Could you check a few things on this model? Use its own coordinates, in mm. Round coordinates to 2 decimals unless told otherwise and drop trailing zeros. Loops run counter-clockwise (first coordinate to the right, second up) from the corner with the lowest first, then second, coordinate; pieces in that order, holes last. Notation, with made-up numbers: (11.5, -38.5) - (37.5, -38.5) arc R15 ccw to (37.5, -22.5) - close; hole circle Ø1 at (-20.75, 47). An arc over 180 degrees is marked (long way). Use one line per item in the form item = value.
```python
from build123d import *

# Parameters (mm, degrees)
F1_DEPTH = 40.64
F3_D     = 22.098
F5_DEPTH = 14.732
F7_DEPTH = 14.732
F9_D     = 13.97


with BuildPart() as f1:
    # F0 (on Right) → F1 (new body)
    with BuildSketch(Plane.YZ):
        with BuildLine():
            Line((68.5798105303, 21.9367931967), (0, 22.098))
            ThreePointArc((0, 22.098), (-22.098, 0), (0, -22.098))
            Line((0, -22.098), (68.5798105303, -22.098))
            Line((68.5798105303, -22.098), (68.5798105303, -7.366))
            Line((68.5798105303, -7.366), (24.1298105303, -7.366))
            Line((24.1298105303, -7.366), (24.1298105303, 7.2047931967))
            Line((24.1298105303, 7.2047931967), (68.5798105303, 7.2047931967))
            Line((68.5798105303, 7.2047931967), (68.5798105303, 21.9367931967))
        make_face()
    extrude(amount=-F1_DEPTH)

    # F3 (through all)
    with Locations(Plane.YZ):
        with Locations((0, 0)):
            Hole(F3_D / 2)

    # F4 (on face) → F5 (join)
    with BuildSketch(Plane(origin=(0, 0.0519442709, 22.0978778974), x_dir=(1, 0, 0), z_dir=(0, 0.0023506387, 0.9999972372))):
        with BuildLine():
            Line((-40.64, 68.5280555856), (0, 68.5280555856))
            ThreePointArc((0, 68.5280555856), (-20.32, 88.8480555856), (-40.64, 68.5280555856))
        make_face()
    extrude(amount=-F5_DEPTH)

    # F6 (on face) → F7 (join)
    with BuildSketch(Plane(origin=(0, 0, -22.098), x_dir=(1, 0, 0), z_dir=(0, 0, -1))):
        with BuildLine():
            ThreePointArc((-40.64, -68.5798105303), (-20.32, -88.8998105303), (0, -68.5798105303))
            Line((0, -68.5798105303), (-40.64, -68.5798105303))
        make_face()
    extrude(amount=-F7_DEPTH)

    # F9 (through all)
    with Locations(Plane(origin=(0, 0, -22.098), x_dir=(1, 0, 0), z_dir=(0, 0, -1))):
        with Locations((-20.32, -68.5798105303)):
            Hole(F9_D / 2)


solid = f1.part
```
1. For P1, Ø4.5, axis at x = -11.5, z = 2, coming from the +Y side; P2, Ø1.5, axis at x = -7, z = 16, coming from the -Y side; P3, Ø22.5, axis at x = -20.32, y = 68.58, coming from the -Z side; P4, Ø6, axis at x = -16.5, z = -4, coming from the -Y side, each with a flat end and sliding along its axis, tell me the tip position at first contact or that it passes through.
Solution:
P1 = 24.13
P2 = -15.99
P3 = -22.1
P4 = -22.08
2. We'd pull the mould along X, two halves only. Please class faces 1 (the face through (-18.81, 75.4, 14.67)), 2 (the face through (-40.64, 23, 0)), 3 (the face through (-18.81, 75.4, -14.63)), 4 (the face through (-20.036, -22.093, 0.486)): +X half, -X half, draft (parallel to the pull), parting line (faces both ways), or undercut.
Solution:
face_1 = undercut
face_2 = -X half
face_3 = undercut
face_4 = draft
3. If we section it at A-A, the plane z = 0: Write out the boundary of the cut face in (x, y).
Solution:
outline = (-40.64, -22.1) - (0, -22.1) - (0, -11.05) - (-40.64, -11.05) - close; (-40.64, 11.05) - (0, 11.05) - (0, 24.13) - (-40.64, 24.13) - close
4. If we section it at D-D, the plane x = -16: Write out the boundary of the cut face in (y, z).
Solution:
outline = (0, -22.1) - (63.09, -22.1) - (63.09, -7.37) - (24.13, -7.37) - (24.13, 7.2) - (63.09, 7.2) - (63.09, 21.95) - (0, 22.1) arc R22.1 ccw to start; (74.07, -22.1) - (88.44, -22.1) - (88.44, -7.37) - (74.07, -7.37) - close; (74.07, 7.19) - (88.4, 7.16) - (88.44, 21.89) - (74.07, 21.92) - close; hole circle Ø22.1 at (0, 0)
5. If we section it at C-C, the plane x = -32.5: Write out the boundary of the cut face in (y, z), plus the area to 3 significant figures.
Solution:
outline = (0, -22.1) - (84.84, -22.1) - (84.84, -7.37) - (24.13, -7.37) - (24.13, 7.2) - (68.56, 7.2) - (84.81, 7.17) - (84.84, 21.9) - (0, 22.1) arc R22.1 ccw to start; hole circle Ø22.1 at (0, 0)
area = 3,240 mm^2
6. Please list where these lines run through material, in increasing order: line 1 along Z through (x, y) = (-36, 67); line 2 along Z through (x, y) = (-3, 54); line 3 along Y through (x, z) = (-23, 2).
Solution:
line_1 = -22.1 to -7.37, 7.2 to 21.94
line_2 = -22.1 to -7.37, 7.2 to 21.97
line_3 = -22.01 to -10.87, 10.87 to 24.13
7. If we section it at B-B, the plane x = -24.5: Write out the boundary of the cut face in (y, z), plus the area to 3 significant figures.
Solution:
outline = (0, -22.1) - (62.98, -22.1) - (62.98, -7.37) - (24.13, -7.37) - (24.13, 7.2) - (62.98, 7.2) - (62.98, 21.95) - (0, 22.1) arc R22.1 ccw to start; (74.18, -22.1) - (88.47, -22.1) - (88.47, -7.37) - (74.18, -7.37) - close; (74.18, 7.19) - (88.43, 7.16) - (88.47, 21.89) - (74.18, 21.92) - close; hole circle Ø22.1 at (0, 0)
area = 3,020 mm^2
